Build history of the part. All positions in model axes, mm. Round coordinates to 2 decimals unless told otherwise and drop trailing zeros. Write each loop counter-clockwise with the first axis right and the second up, starting at its lowest first coordinate (ties: lowest second). Pieces come first, ordered by that corner, then holes.
Item 1: Band-saw the part on B-B, the plane z = 18.5. Write the cut outline in (x, y).
Item 2: Band-saw the part on A-A, the plane y = -41.5. Write the cut outline in (x, z).
Item 3: Wall check: probe 1 along X at (y, z) = (-51.5, 22.5); probe 2 along X at (y, z) = (34, -29.5); probe 3 along X at (y, z) = (-64.5, -31.5). Give the ranges that are in metal, low to high.
Item 4: Drop flat-ended pins along their axis: pin 1 Ø1 at (x, y) = (8, 21) entering from -Z; pin 2 Ø1 at (y, z) = (12.5, 32) entering from +X; pin 3 Ø2 at (x, y) = (-1, -50) entering from -Z; pin 4 Ø11 at (x, z) = (-0.5, 22.5) entering from +Y. Give the stop position or say it passes through.
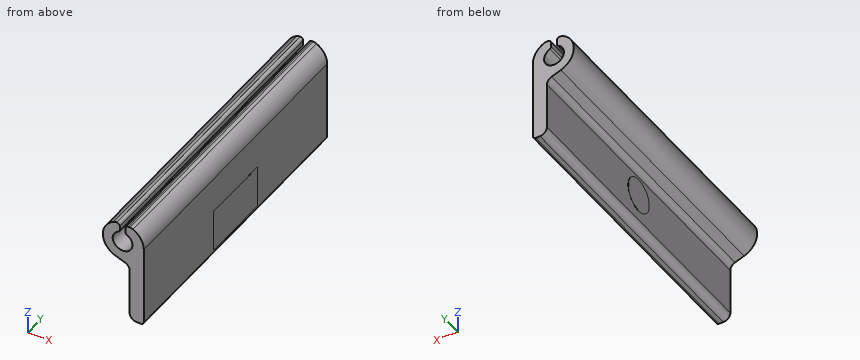
```python
from build123d import *

# Parameters (mm, degrees)
F1_DEPTH = 105
F2_R     = 12
F3_DEPTH = 0.05
F4_W     = 50
F4_H     = 30
F5_DEPTH = 0.01


# Not quite as in the source:
# - ends of sketch curves that miss each other by under 0.0002 mm in the source are joined


with BuildPart() as f1:
    # F0 (on Front) → F1 (new body, symmetric)
    with BuildSketch(Plane.XZ):
        with BuildLine():
            Line((4.4999999997, -23.5), (4.4999999997, -30.5))
            ThreePointArc((4.4999999997, -30.5), (5.9644660938, -34.0355339059), (9.4999999997, -35.5))
            Line((9.4999999997, -35.5), (12.5, -35.5))
            ThreePointArc((12.5, -35.5), (13.9142133287, -34.9142135624), (14.4999997663, -33.5))
            Line((14.4999997663, -33.5), (14.4999997663, 22.4999994828))
            ThreePointArc((14.4999997663, 22.4999994828), (12.4539129776, 29.7872458033), (6.9137199183, 34.9444437777))
            ThreePointArc((6.9137199183, 34.9444437777), (5.8016169865, 35.3591259101), (4.6231056877, 35.4999993303))
            Line((4.6231056877, 35.4999993303), (3.4999997663, 35.4999993303))
            ThreePointArc((3.4999997663, 35.4999993303), (2.0857862039, 34.9142128927), (1.4999997663, 33.4999993303))
            Line((1.4999997663, 33.4999993303), (1.4999997663, 30.2459664828))
            ThreePointArc((1.4999997663, 30.2459664828), (1.7397477835, 29.4324771221), (2.3823530195, 28.8790310431))
            ThreePointArc((2.3823530195, 28.8790310431), (-0.5000000985, 15.4999997293), (-3.3823532363, 28.8790310342))
            ThreePointArc((-3.3823532363, 28.8790310342), (-2.7397478169, 29.4324771961), (-2.4999997997, 30.2459665567))
            Line((-2.4999997997, 30.2459665567), (-2.4999997997, 33.5))
            ThreePointArc((-2.4999997997, 33.5), (-3.0857862373, 34.9142132361), (-4.4999997997, 35.4999996738))
            Line((-4.4999997997, 35.4999996738), (-4.6231058319, 35.4999996738))
            ThreePointArc((-4.6231058319, 35.4999996738), (-5.8016171306, 35.3591262536), (-6.9137200625, 34.9444441212))
            ThreePointArc((-6.9137200625, 34.9444441212), (-14.4718653147, 21.6128794539), (-5.288282, 9.344303))
            Line((-5.288282, 9.344303), (1.210101, 6.979085))
            ThreePointArc((1.210101, 6.979085), (3.5957603078, 5.1485040574), (4.4999999997, 2.2806219993))
            Line((4.4999999997, 2.2806219993), (4.4999999997, 0.5))
            Line((4.4999999997, 0.5), (4.4999999997, -23.5))
        make_face()
    extrude(amount=F1_DEPTH, both=True)

    # F2 (on face) → F3 (join)
    with BuildSketch(Plane(origin=(4.4999999997, 0, 0), x_dir=(0, -1, 0), z_dir=(-1, 0, 0))):
        with Locations((0, -11.5)):
            Circle(F2_R)
    extrude(amount=F3_DEPTH)

    # F4 (on face) → F5 (join)
    with BuildSketch(Plane.YZ.offset(14.4999997663)):
        with Locations((0, -17.5000005172)):
            Rectangle(F4_W, F4_H)
    extrude(amount=F5_DEPTH)


solid = f1.part
```
Results:
1. outline: (-13.92, -105) - (-6.24, -105) - (-6.24, 105) - (-13.92, 105) - close; (5.24, -105) - (14.5, -105) - (14.5, 105) - (5.24, 105) - close
2. outline: (-6.91, 34.94) arc R14 ccw to (-5.29, 9.34) - (1.21, 6.98) arc R5 cw to (4.5, 2.28) - (4.5, -30.5) arc R5 ccw to (9.5, -35.5) - (12.5, -35.5) arc R2 ccw to (14.5, -33.5) - (14.5, 22.5) arc R14 ccw to (6.91, 34.94) arc R5 ccw to (4.62, 35.5) - (3.5, 35.5) arc R2 ccw to (1.5, 33.5) - (1.5, 30.25) arc R1.5 ccw to (2.38, 28.88) arc R7 cw (long way) to (-3.38, 28.88) arc R1.5 ccw to (-2.5, 30.25) - (-2.5, 33.5) arc R2 ccw to (-4.5, 35.5) - (-4.62, 35.5) arc R5 ccw to start
3. probe 1: x = -14.5 to -7.5, 6.5 to 14.5
3. probe 2: x = 4.5 to 14.5
3. probe 3: x = 4.6 to 14.5
4. pin 1: stops at z = -35.4
4. pin 2: stops at x = 11.22
4. pin 3: stops at z = 7.42
4. pin 4: passes through
